```python
from build123d import *

# Parameters (mm, degrees)
F2_SIZE = 0.4


with BuildPart() as f1:
    # F0 (on Front) → F1 (revolve)
    with BuildSketch(Plane.XZ):
        Polygon((3.5, 3), (3.5, 0), (8.231808, 0), (8.231808, 0.431463), (6.11, 1), (6.11, 8.5), (8.231808, 9.068537), (8.231808, 9.5), (3.5, 9.5), (3.5, 6.5), (1.6, 6.5), (1.6, 3), align=None)
    revolve(axis=Axis((0, 0, 7.577015), (0, 0, 1)))

    # F2
    f2_edges = [f1.edges().sort_by_distance(p)[0] for p in [
        (-3.5, 0, 9.5),
        (-3.5, 0, 0),
        (-1.6, 0, 6.5),
        (-1.6, 0, 3),
        (1.6, 0, 4.75),
    ]]
    chamfer(f2_edges, length=F2_SIZE)


solid = f1.part
```
The listing builds one solid part. Answer for the finished solid, in the listing's coordinates (mm). A direction names the side the tool comes from. Give positions to 0.01 mm unless a question says otherwise; leave off trailing zeros. Write each loop counter-clockwise with the first axis right and the second up, starting at its lowest first coordinate (ties: lowest second). Pieces come first, ordered by that corner, then holes. Notation, with made-up numbers: (0, 71.25) - (10, 71.25) arc R18 cw to (10, 91.25) - close; hole circle Ø3 at (69, -0.75). An arc over 180 degrees is marked (long way). Use one line per item in the form item = value. Start each with the question number.
1) The mould has two halves that part along Y. Classify faces 4 (the face through (3.233, -1.341, 7.782)), 5 (the face through (5.828, 1.835, 4.802)), 6 (the face through (-2, -4, 0)), 7 (the face through (3.233, -1.341, 1.682)): pulls with the +Y half, pulls with the -Y half, needs draft (parallel to the pull), parting line crosses it, or undercut.
2) A tool of negligible diameter and unlimited length cuts with its end or side. For faces 1 (the face through (-2, -2, 3)), 2 (the face through (2, -4, 9.5)), 3 (the face through (2, -2, 6.5)), from which of +Z, -Z, +X, -X, +Y, -Y can it reach the whole face along a straight path? Write none if from no direction.
3) Find section D-D on z = 5. Determine the outline of the cut face in (x, y).
4) Find section C-C on z = 2.75. Determine the outline of the cut face in (x, y).
5) Consider line 1 along Y through (x, z) = (0, 7.85); line 2 along Z through (x, y) = (1, 2.25); line 3 along Y through (x, z) = (-2.25, 1.5). Determine where each line is inside the solid, lowest interval first. Write a range as from..to.
6) Flat-ended cylindrical pins translate along their axes: pin 1 Ø4 at (x, z) = (2.5, 4.5) entering from -Y; pin 2 Ø4 at (y, z) = (-6, 4) entering from -X; pin 3 Ø3 at (y, z) = (0, 5.5) entering from -X. Find the tip coordinate at first contact, or state that the pin passes through.
Geometry results:
q1.face_4 = undercut
q1.face_5 = parting line crosses it
q1.face_6 = needs draft
q1.face_7 = undercut
q2.face_1 = -Z
q2.face_2 = +Z, +X, -X, +Y, -Y
q2.face_3 = +Z
q3.outline = circle Ø12.22 at (0, 0); hole circle Ø3.2 at (0, 0)
q4.outline = circle Ø12.22 at (0, 0); hole circle Ø7 at (0, 0)
q5.line_1 = -6.11..-3.5, 3.5..6.11
q5.line_2 = 3..6.5
q5.line_3 = -5.68..-2.68, 2.68..5.68
q6.pin_1 = -6.09
q6.pin_2 = -4.62
q6.pin_3 = -6.11
